Part model, mm, in its own coordinate system. Give positions to 0.01 mm unless a question says otherwise; leave off trailing zeros. Loops run counter-clockwise (first coordinate to the right, second up) from the corner with the lowest first, then second, coordinate; pieces in that order, holes last. Notation, with made-up numbers: (34.25, 72) -> (66.25, 72) arc R20 ccw to (66.25, 88) -> close; hole circle Ø9 at (17.5, -33). An arc over 180 degrees is marked (long way). One line per question, with ' | ' between items.
```python
from build123d import *

# Parameters (mm, degrees)
F0_W           = 127
F0_H           = 152.4
F1_DEPTH       = 9
F3_D           = 9
F5_D           = 6.6
F5_CBORE_D     = 11.25
F5_CBORE_DEPTH = 6
F6_R           = 5.08


with BuildPart() as f1:
    # F0 (on Front) → F1 (new body)
    with BuildSketch(Plane.XZ):
        Rectangle(F0_W, F0_H)
    extrude(amount=F1_DEPTH)

    # F3 (through all)
    with Locations(Plane.XZ.offset(9)):
        with Locations((0, 65), (0, -65)):
            Hole(F3_D / 2)

    # F5 (through all)
    with Locations(Plane.XZ.offset(9)):
        with Locations((-50, 50), (50, 50), (50, -50), (-50, -50)):
            CounterBoreHole(F5_D / 2, F5_CBORE_D / 2, F5_CBORE_DEPTH)

    # F6
    f6_edges = [f1.edges().sort_by_distance(p)[0] for p in [
        (63.5, -4.5, 76.2),
        (63.5, -4.5, -76.2),
        (-63.5, -4.5, -76.2),
        (-63.5, -4.5, 76.2),
    ]]
    fillet(f6_edges, radius=F6_R)


solid = f1.part
```
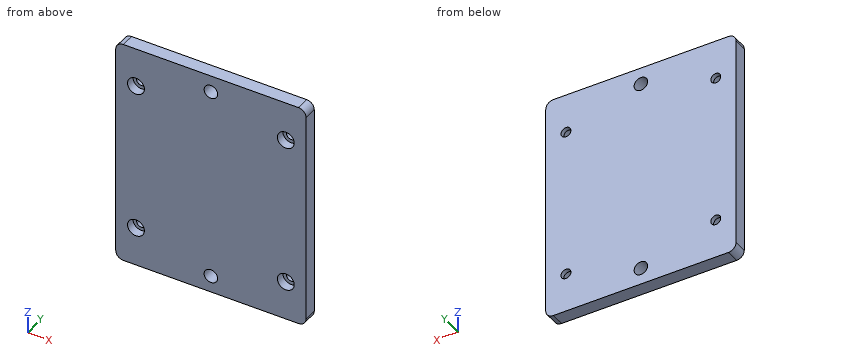
1) Saw through at C-C (z = 65). Give the cut face in (x, y).
Found:
outline: (-63.5, -9) -> (-4.5, -9) -> (-4.5, 0) -> (-63.5, 0) -> close; (4.5, -9) -> (63.5, -9) -> (63.5, 0) -> (4.5, 0) -> close
2) Drill centre lines: line 1 (Z direction, x = 50, y = -1.9); line 2 (Z direction, x = 0, y = -2); line 3 (X direction, y = -7, z = -49). Where is each one in solid material? Low to high.
Found:
line 1: -76.2 to -53.3, -46.7 to 46.7, 53.3 to 76.2 | line 2: -76.2 to -69.5, -60.5 to 60.5, 69.5 to 76.2 | line 3: -63.5 to -55.54, -44.46 to 44.46, 55.54 to 63.5
3) Saw through at B-B (x = 0). Give the cut face in (y, z).
Found:
outline: (-9, -76.2) -> (0, -76.2) -> (0, -69.5) -> (-9, -69.5) -> close; (-9, -60.5) -> (0, -60.5) -> (0, 60.5) -> (-9, 60.5) -> close; (-9, 69.5) -> (0, 69.5) -> (0, 76.2) -> (-9, 76.2) -> close
4) Saw through at A-A (y = -6.75). Give the cut face in (x, z) (3 decimals).
Found:
outline: (-63.5, -71.12) arc R5.08 ccw to (-58.42, -76.2) -> (58.42, -76.2) arc R5.08 ccw to (63.5, -71.12) -> (63.5, 71.12) arc R5.08 ccw to (58.42, 76.2) -> (-58.42, 76.2) arc R5.08 ccw to (-63.5, 71.12) -> close; hole circle Ø11.25 at (-50, -50); hole circle Ø11.25 at (-50, 50); hole circle Ø9 at (0, -65); hole circle Ø9 at (0, 65); hole circle Ø11.25 at (50, -50); hole circle Ø11.25 at (50, 50)
5) Pin check, flat tips, straight feed: P1, Ø9, axis at x = -51.5, z = 49.5, coming from the -Y side; P2, Ø9, axis at x = 50, z = 50, coming from the -Y side; P3, Ø7, axis at x = 0, z = 65, coming from the +Y side. Stop position of each tip, or through.
Found:
P1: y = -9 | P2: y = -3 | P3: through
6) Saw through at D-D (x = -50). Give the cut face in (y, z) (3 decimals), and give its area (3 significant figures).
Found:
outline: (-9, -76.2) -> (0, -76.2) -> (0, -53.3) -> (-3, -53.3) -> (-3, -55.625) -> (-9, -55.625) -> close; (-9, -44.375) -> (-3, -44.375) -> (-3, -46.7) -> (0, -46.7) -> (0, 46.7) -> (-3, 46.7) -> (-3, 44.375) -> (-9, 44.375) -> close; (-9, 55.625) -> (-3, 55.625) -> (-3, 53.3) -> (0, 53.3) -> (0, 76.2) -> (-9, 76.2) -> close | area: 1,200 mm2
